Autodesk Inventor part; units mm, degrees
ref_plane "Work Plane1" through (1.525, 0, 0) normal (0, 0, 1) x (1, 0, 0)
ref_plane "Work Plane2" through (-2.5005, 0, 0) normal (1, 0, 0) x (0, 0, -1)
ref_plane "YZ Plane" through (0, 0, 0) normal (1, 0, 0) x (0, 1, 0)
sketch "Sketch1" plane through (0, 0, 0) normal (0, 0, 1) x (1, 0, 0)
  line L0 (0, 2.5) -> (0, 1.25)
  line L1 (1.3, 1.25) -> (6, 1.25)
  line L2 (6, 1.25) -> (6, 0)
  line L3 (6, 0) -> (-0.0011, 0)
  line L4 (-1.2013, 0) -> (7.2002, 0)
  line L5 (-0.0011, 0) -> (-0.0011, 2.5)
  line L6 (-0.0011, 2.5) -> (0, 2.5)
  line L7 (1.3, 1.25) -> (1.0238, 1.25)
  line L8 (1.0238, 1.25) -> (0, 1.25)
  line L9 (0, -0.5) -> (0, 3)
  dimension "d0" = 6
  dimension "d1" = 4.7
  dimension "d2" = 2.5
  dimension "d9" = 0.0011
  dimension "d10" = 5
  dimension "d13" = 0.2762
  dimension "d14" = 2.5
revolve "Body" add sketch "Sketch1" angle 360 about axis through (6, 0, 0) along (-1, 0, 0)
sketch "Sketch2" plane through (-0.0011, 0, 0) normal (-1, 0, 0) x (0, 0, 1)
  line L0 (0, 2.8868) -> (2.5, 1.4434)
  line L1 (2.5, 1.4434) -> (2.5, -1.4434)
  line L2 (2.5, -1.4434) -> (0, -2.8868)
  line L3 (0, -2.8868) -> (-2.5, -1.4434)
  line L4 (-2.5, -1.4434) -> (-2.5, 1.4434)
  line L5 (-2.5, 1.4434) -> (0, 2.8868)
  point P0 (0, 0)
  point P1 (0, 0)
  dimension "d11" = 5
extrude "Head" add sketch "Sketch2" along normal blind 5
sketch "Sketch4" plane through (0, 0, 0) normal (0, 0, 1) x (1, 0, 0)
  line L0 (-5.0011, 2.5) -> (-5.0011, 2.8868)
  line L1 (-5.0011, 2.8868) -> (-4.7778, 2.8868)
  line L2 (-4.7778, 2.8868) -> (-5.0011, 2.5)
  line L3 (-2.0399, 0) -> (0.3387, 0)
  line L4 (-0.0011, 2.8868) -> (-5.0011, 2.8868)
  line L5 (-5.0011, 1.4434) -> (-5.0011, 2.8868)
  line L6 (-0.0011, -2.8868) -> (-5.0011, -2.8868)
  line L7 (-0.0011, 2.1651) -> (-0.0011, 2.8868)
  line L8 (-0.0011, 2.8868) -> (-0.2244, 2.8868)
  dimension "d5" = 30
  dimension "d19" = 5
revolve "Chamfer1" cut sketch "Sketch4" angle 360 about axis through (-10, 0, 0) along (1, 0, 0)
thread "Thread"
chamfer "Chamfer2" distance 0.2761 distance2 0.2762 1 edges at (6, -1.25, 0) measured on face at (6, -0.3871, 0.3429)
ref_plane "Work Plane1" through (1.525, 0, 0) normal (0, 0, 1) x (1, 0, 0)
sketch "Sketch7" plane through (-5.0011, 0, 0) normal (-1, 0, 0) x (0, 0, 1)
  circle A0 centre (0, 0) radius 1.45
  point P0 (0, 0)
  dimension "d59" = 2.9
extrude "Extrusion5" cut sketch "Sketch7" against normal blind 20
ref_plane "Work Plane2" through (-2.5005, 0, 0) normal (1, 0, 0) x (0, 0, -1)
mirror "Mirror1" about plane through (-2.5005, 0, 0) normal (1, 0, 0) of "Chamfer1"
equation "\"d11\" = SW"
equation "\"d15\" = GEL"
equation "\"d6\" = -0.5 * SPD + 0.5 * GD"
equation "\"d0\" = NLG"
equation "\"d1\" = GEL"
equation "\"d2\" = GD"
equation "\"d10\" = SD2"
equation "\"d14\" = BDM"
equation "\"d5\" = ANG1"
equation "\"d19\" = SW0"
equation "\"NLG\" = 6"
equation "\"GD\" = NND"
equation "\"BDM\" = NND"
equation "\"KOH\" = 1.7"
equation "\"GEL\" = 4.7"
equation "\"SW\" = 5"
equation "\"SW0\" = SW"
equation "\"SPD\" = NND - 1.2269 * PTC"
equation "\"SD2\" = SW"
equation "\"SD\" = 0.001"
equation "\"ANG1\" = 30deg"
equation "\"GAL\" = 0.61345 * PTC"
equation "\"GUL\" = 0.61345 * PTC"
equation "\"RR\" = 0.001"
equation "\"WFT\" = SD"
equation "\"GD1\" = THREADDIA - 1.2269 * PTC"
equation "\"THREADDIA\" = 2.5"
equation "\"SDH\" = SW"
equation "\"TOA\" = 30deg"
equation "\"FAWI\" = 45deg"
equation "\"PTC\" = 0.45"
equation "\"NND\" = 2.5"
equation "\"E0\" = 1.155 * SW"
properties part number "AS 1110 - M2.5 x 6" material "Steel, Mild"
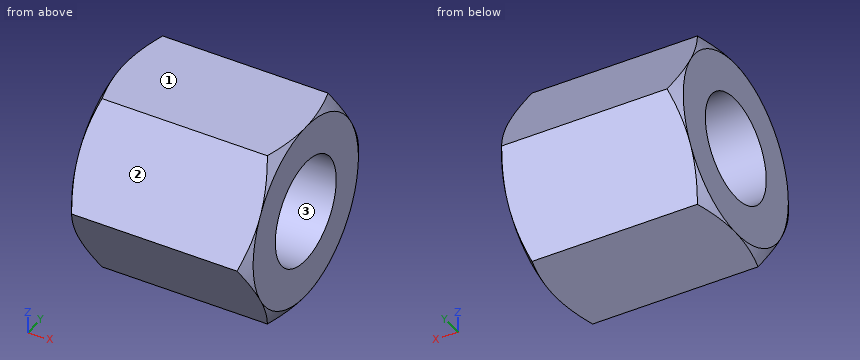
Could you check a few things on this model? Use its own coordinates, in mm. Face numbers are marked on the shaded views. Round coordinates to 2 decimals unless told otherwise and drop trailing zeros. Loops run counter-clockwise (first coordinate to the right, second up) from the corner with the lowest first, then second, coordinate; pieces in that order, holes last.
Q1. I want a section at A-A (x = -2.5). Write out the boundary of the cut face in (y, z).
Q2. Thinking about a two-plate mould opening in Y: for the marked faces 1, 2 and 3, which applies, pulls with the +Y half, pulls with the -Y half, needs draft (parallel to the pull), parting line crosses it, or undercut?
Q3. For P1, Ø1, axis at x = -2, z = -1.5, coming from the -Y side; P2, Ø1.5, axis at x = -2.5, y = 2.5, coming from the -Z side; P3, Ø1, axis at y = 0.5, z = 0, coming from the +X side, each with a flat end and sliding along its axis, tell me the tip position at first contact or that it passes through.
Q4. Please list where these lines run through material, in increasing order: L1, parallel to Y at x = -3.1, z = -1.3; L2, parallel to Z at x = -0.9, y = -1.2; L3, parallel to Z at x = -4.05, y = 1.1.
Answer below:
1. outline: (-2.89, 0) - (-1.44, -2.5) - (1.44, -2.5) - (2.89, 0) - (1.44, 2.5) - (-1.44, 2.5) - close; hole circle Ø2.9 at (0, 0)
2. face 1: needs draft
2. face 2: pulls with the -Y half
2. face 3: undercut
3. P1: stops at y = -2.31
3. P2: stops at z = -1.97
3. P3: passes through
4. L1: y = -2.14 to -0.64, 0.64 to 2.14
4. L2: z = -2.5 to -0.81, 0.81 to 2.5
4. L3: z = -2.5 to -0.94, 0.94 to 2.5
